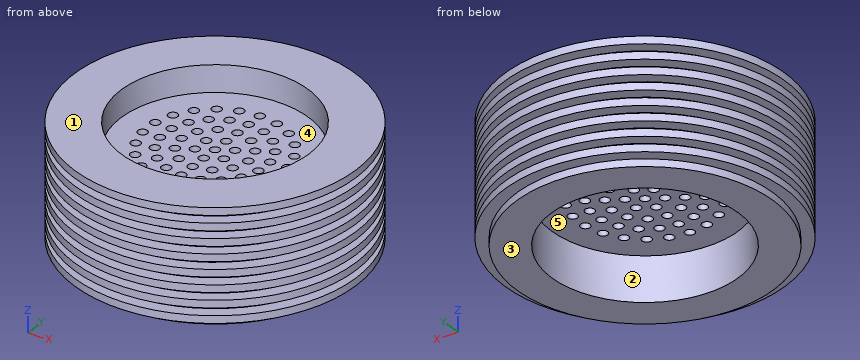
from build123d import *

# Parameters (mm, degrees)
ESQUISSE1_R                = 38.1
BOSS_EXTRU_1_DEPTH         = 32
ESQUISSE2_R                = 25.4
ENL_V_MAT_EXTRU_1_DEPTH    = 12.1
ESQUISSE3_R                = 1.3
ENL_V_MAT_EXTRU_2_DEPTH    = 12.7
ESQUISSE4_R                = 25.4
ENL_V_MAT_EXTRU_3_DEPTH    = 60.314922237
ESQUISSE5_OUTSIDE_W        = 100.682
ESQUISSE5_OUTSIDE_H        = 100.682
ESQUISSE5_OUTSIDE_R        = 34.925
ENL_V_MAT_EXTRU_4_DEPTH    = 2
R_P_TITION_LIN_AIRE1_COUNT = 8
R_P_TITION_LIN_AIRE1_PITCH = 4


with BuildPart() as part:
    # Esquisse1 → Boss.-Extru.1 (new body)
    with BuildSketch(Plane.XY):
        Circle(ESQUISSE1_R)
    extrude(amount=BOSS_EXTRU_1_DEPTH)

    # Esquisse2 → Enlèv. mat.-Extru.1 (cut)
    with BuildSketch(Plane(origin=(0, 0, 0), x_dir=(-1, 0, 0), z_dir=(0, 0, -1))):
        Circle(ESQUISSE2_R)
    extrude(amount=-ENL_V_MAT_EXTRU_1_DEPTH, mode=Mode.SUBTRACT)

    # Esquisse3 → Enlèv. mat.-Extru.2 (cut)
    with BuildSketch(Plane(origin=(0, 0, 12.1), x_dir=(-1, 0, 0), z_dir=(0, 0, -1))):
        Circle(ESQUISSE3_R)
        with Locations((0, 4.5)):
            Circle(ESQUISSE3_R)
        with Locations((0, 9)):
            Circle(ESQUISSE3_R)
        with Locations((0, 13.5)):
            Circle(ESQUISSE3_R)
        with Locations((0, 18)):
            Circle(ESQUISSE3_R)
        with Locations((3.897114317, 2.25)):
            Circle(ESQUISSE3_R)
        with Locations((3.897114317, -2.25)):
            Circle(ESQUISSE3_R)
        with Locations((0, -4.5)):
            Circle(ESQUISSE3_R)
        with Locations((-3.897114317, -2.25)):
            Circle(ESQUISSE3_R)
        with Locations((-3.897114317, 2.25)):
            Circle(ESQUISSE3_R)
        with Locations((4.5, 7.794228634)):
            Circle(ESQUISSE3_R)
        with Locations((7.794228634, 4.5)):
            Circle(ESQUISSE3_R)
        with Locations((9, 0)):
            Circle(ESQUISSE3_R)
        with Locations((7.794228634, -4.5)):
            Circle(ESQUISSE3_R)
        with Locations((4.5, -7.794228634)):
            Circle(ESQUISSE3_R)
        with Locations((0, -9)):
            Circle(ESQUISSE3_R)
        with Locations((-4.5, -7.794228634)):
            Circle(ESQUISSE3_R)
        with Locations((-7.794228634, -4.5)):
            Circle(ESQUISSE3_R)
        with Locations((-9, 0)):
            Circle(ESQUISSE3_R)
        with Locations((-7.794228634, 4.5)):
            Circle(ESQUISSE3_R)
        with Locations((-4.5, 7.794228634)):
            Circle(ESQUISSE3_R)
        with Locations((4.617271935, 12.685850381)):
            Circle(ESQUISSE3_R)
        with Locations((8.677632731, 10.341599982)):
            Circle(ESQUISSE3_R)
        with Locations((11.691342951, 6.75)):
            Circle(ESQUISSE3_R)
        with Locations((13.294904666, 2.344250399)):
            Circle(ESQUISSE3_R)
        with Locations((13.294904666, -2.344250399)):
            Circle(ESQUISSE3_R)
        with Locations((11.691342951, -6.75)):
            Circle(ESQUISSE3_R)
        with Locations((8.677632731, -10.341599982)):
            Circle(ESQUISSE3_R)
        with Locations((4.617271935, -12.685850381)):
            Circle(ESQUISSE3_R)
        with Locations((0, -13.5)):
            Circle(ESQUISSE3_R)
        with Locations((-4.617271935, -12.685850381)):
            Circle(ESQUISSE3_R)
        with Locations((-8.677632731, -10.341599982)):
            Circle(ESQUISSE3_R)
        with Locations((-11.691342951, -6.75)):
            Circle(ESQUISSE3_R)
        with Locations((-13.294904666, -2.344250399)):
            Circle(ESQUISSE3_R)
        with Locations((-13.294904666, 2.344250399)):
            Circle(ESQUISSE3_R)
        with Locations((-11.691342951, 6.75)):
            Circle(ESQUISSE3_R)
        with Locations((-8.677632731, 10.341599982)):
            Circle(ESQUISSE3_R)
        with Locations((-4.617271935, 12.685850381)):
            Circle(ESQUISSE3_R)
        with Locations((5.071186023, 17.270873525)):
            Circle(ESQUISSE3_R)
        with Locations((9.731534714, 15.142563591)):
            Circle(ESQUISSE3_R)
        with Locations((13.603492338, 11.787493211)):
            Circle(ESQUISSE3_R)
        with Locations((16.373375916, 7.477470234)):
            Circle(ESQUISSE3_R)
        with Locations((17.816785954, 2.561667089)):
            Circle(ESQUISSE3_R)
        with Locations((17.816785954, -2.561667089)):
            Circle(ESQUISSE3_R)
        with Locations((16.373375916, -7.477470234)):
            Circle(ESQUISSE3_R)
        with Locations((13.603492338, -11.787493211)):
            Circle(ESQUISSE3_R)
        with Locations((9.731534714, -15.142563591)):
            Circle(ESQUISSE3_R)
        with Locations((5.071186023, -17.270873525)):
            Circle(ESQUISSE3_R)
        with Locations((0, -18)):
            Circle(ESQUISSE3_R)
        with Locations((-5.071186023, -17.270873525)):
            Circle(ESQUISSE3_R)
        with Locations((-9.731534714, -15.142563591)):
            Circle(ESQUISSE3_R)
        with Locations((-13.603492338, -11.787493211)):
            Circle(ESQUISSE3_R)
        with Locations((-16.373375916, -7.477470234)):
            Circle(ESQUISSE3_R)
        with Locations((-17.816785954, -2.561667089)):
            Circle(ESQUISSE3_R)
        with Locations((-17.816785954, 2.561667089)):
            Circle(ESQUISSE3_R)
        with Locations((-16.373375916, 7.477470234)):
            Circle(ESQUISSE3_R)
        with Locations((-13.603492338, 11.787493211)):
            Circle(ESQUISSE3_R)
        with Locations((-9.731534714, 15.142563591)):
            Circle(ESQUISSE3_R)
        with Locations((-5.071186023, 17.270873525)):
            Circle(ESQUISSE3_R)
    extrude(amount=-ENL_V_MAT_EXTRU_2_DEPTH, mode=Mode.SUBTRACT)

    # Esquisse4 → Enlèv. mat.-Extru.3 (cut, through all)
    with BuildSketch(Plane(origin=(0, 0, 24.8), x_dir=(-1, 0, 0), z_dir=(0, 0, -1))):
        Circle(ESQUISSE4_R)
    extrude(amount=-ENL_V_MAT_EXTRU_3_DEPTH, mode=Mode.SUBTRACT)

    # Esquisse5 outside → Enlèv. mat.-Extru.4 (cut)
    with BuildSketch(Plane(origin=(0, 0, 0), x_dir=(-1, 0, 0), z_dir=(0, 0, -1))):
        Rectangle(ESQUISSE5_OUTSIDE_W, ESQUISSE5_OUTSIDE_H)
        Circle(ESQUISSE5_OUTSIDE_R, mode=Mode.SUBTRACT)
    enl_v_mat_extru_4 = extrude(amount=-ENL_V_MAT_EXTRU_4_DEPTH, mode=Mode.SUBTRACT)

    # Répétition linéaire1: Enlèv. mat.-Extru.4 ×8
    with Locations(*[(0, 0, i * R_P_TITION_LIN_AIRE1_PITCH) for i in range(1, R_P_TITION_LIN_AIRE1_COUNT)]):
        add(enl_v_mat_extru_4, mode=Mode.SUBTRACT)


solid = part.part
Work out the finished part from the listing and answer in its coordinate system (mm). Face numbers are marked on the shaded views. A direction names the side the tool comes from. Give positions to 0.01 mm unless a question says otherwise; leave off trailing zeros. Order: outer loops, then holes, each group sorted by start corner. A loop starts at its lowest first (then second) coordinate and runs counter-clockwise, first axis right, second up. Notation, with made-up numbers: (65, 33.5) -> (116, 33.5) arc R11 cw to (116, 44.5) -> close; hole circle Ø3 at (87, -11.75). An arc over 180 degrees is marked (long way). Answer as a JSON object with one key per item and string values. Group by question number.
1. The mould has two halves that part along Y. Classify the marked faces 1 and 2: released by +Y, released by -Y, zero draft, split by the parting line, or undercut.
2. Section A-A on x = 0 is taken. Count the separate pieces of the cut face and the enclosed holes in it, plus the area to 3 significant figures.
3. Consider line 1 along Z through (x, y) = (11, 9.5); line 2 along Y through (x, z) = (-14, 17); line 3 along X through (y, z) = (4, 17). Determine where each line is inside the solid, lowest interval first. Write a range as [from, to].
4. Section B-B on z = 29 is taken. Determine the outline of the cut face in (x, y) (3 decimals), plus the area to 3 significant figures.
5. Flat-ended cylindrical pins translate along their axes: pin 1 Ø10 at (x, y) = (0, -12) entering from -Z; pin 2 Ø3 at (x, z) = (23.5, 10) entering from +Y; pin 3 Ø2.5 at (x, y) = (17.82, -2.56) entering from -Z; pin 4 Ø3 at (y, z) = (-8, 26.5) entering from +X. Find the tip coordinate at first contact, or state that the pin passes through.
6. A tool of negligible diameter and unlimited length cuts with its end or side. For the marked faces 3, 4 and 5, from which of +Z, -Z, +X, -X, +Y, -Y can it reach the whole face along a straight path? Write none if from no direction.
7. Section D-D on z = 3 is taken. Determine the outline of the cut face in (x, y), plus the area to 3 significant figures.
Result sheet:
{
 "1": {"face 1": "zero draft", "face 2": "undercut"},
 "2": {"separate pieces": "10", "enclosed holes": "0", "area": "1,060 mm^2"},
 "3": {"line 1": "z = [12.1, 24.8]", "line 2": "y = [-32, -13.03], [-10.55, -3.44], [-1.25, 1.25], [3.44, 10.55], [13.03, 32]", "line 3": "x = [-34.7, -8.99], [-6.59, -1.2], [1.2, 6.59], [8.99, 34.7]"},
 "4": {"outline": "circle Ø69.85 at (0, 0); hole circle Ø50.8 at (0, 0)", "area": "1,810 mm^2"},
 "5": {"pin 1": "stops at z = 12.1", "pin 2": "stops at y = 31.11", "pin 3": "passes through", "pin 4": "stops at x = 37.54"},
 "6": {"face 3": "-Z, +X, -X, +Y, -Y", "face 4": "+Z", "face 5": "-Z"},
 "7": {"outline": "circle Ø76.2 at (0, 0); hole circle Ø50.8 at (0, 0)", "area": "2,530 mm^2"}
}
